Autodesk Fusion 360 part; units mm, degrees
sketch "center" plane through (0, 0, 0) normal (0, 0, 1) x (1, 0, 0)
  line L0 (3.9767, 19.6007) -> (11, 21)
  line L1 (11, 21) -> (9.3026, 17.7049)
  arc A0 (3.9767, 19.6007) -> (0, 20) centre (0, 0) ccw
  arc A1 (11.8706, 16.0962) -> (9.3026, 17.7049) centre (0, 0) ccw
  arc A2 (-8.3037, 18.1947) -> (-11.7557, 16.1803) centre (0, 0) ccw
  line L2 (-8.3037, 18.1947) -> (-3.4443, 23.455)
  line L3 (-3.4443, 23.455) -> (-2.8807, 19.7915)
  arc A3 (0.1424, 19.9995) -> (-2.8807, 19.7915) centre (0, 0) ccw
  arc A4 (-17.4124, 9.839) -> (-19.0211, 6.1803) centre (0, 0) ccw
  line L4 (-17.4124, 9.839) -> (-16.573, 16.951)
  line L5 (-16.573, 16.951) -> (-13.9637, 14.3184)
  arc A5 (-11.6402, 16.2636) -> (-13.9637, 14.3184) centre (0, 0) ccw
  arc A6 (-19.8702, -2.2748) -> (-19.0211, -6.1803) centre (0, 0) ccw
  line L6 (-19.8702, -2.2748) -> (-23.3714, 3.9723)
  line L7 (-23.3714, 3.9723) -> (-19.713, 3.3762)
  arc A7 (-18.9766, 6.3156) -> (-19.713, 3.3762) centre (0, 0) ccw
  arc A8 (-14.7382, -13.5198) -> (-11.7557, -16.1803) centre (0, 0) ccw
  line L8 (-14.7382, -13.5198) -> (-21.2427, -10.5237)
  line L9 (-21.2427, -10.5237) -> (-17.9326, -8.8556)
  arc A9 (-19.0647, -6.0447) -> (-17.9326, -8.8556) centre (0, 0) ccw
  arc A10 (-3.9767, -19.6007) -> (0, -20) centre (0, 0) ccw
  line L10 (-3.9767, -19.6007) -> (-11, -21)
  line L11 (-11, -21) -> (-9.3026, -17.7049)
  arc A11 (-11.8706, -16.0962) -> (-9.3026, -17.7049) centre (0, 0) ccw
  arc A12 (8.3037, -18.1947) -> (11.7557, -16.1803) centre (0, 0) ccw
  line L12 (8.3037, -18.1947) -> (3.4443, -23.455)
  line L13 (3.4443, -23.455) -> (2.8807, -19.7915)
  arc A13 (-0.1424, -19.9995) -> (2.8807, -19.7915) centre (0, 0) ccw
  arc A14 (17.4124, -9.839) -> (19.0211, -6.1803) centre (0, 0) ccw
  line L14 (17.4124, -9.839) -> (16.573, -16.951)
  line L15 (16.573, -16.951) -> (13.9637, -14.3184)
  arc A15 (11.6402, -16.2636) -> (13.9637, -14.3184) centre (0, 0) ccw
  arc A16 (19.8702, 2.2748) -> (19.0211, 6.1803) centre (0, 0) ccw
  line L16 (19.8702, 2.2748) -> (23.3714, -3.9723)
  line L17 (23.3714, -3.9723) -> (19.713, -3.3762)
  arc A17 (18.9766, -6.3156) -> (19.713, -3.3762) centre (0, 0) ccw
  arc A18 (14.7382, 13.5198) -> (11.7557, 16.1803) centre (0, 0) ccw
  line L18 (14.7382, 13.5198) -> (21.2427, 10.5237)
  line L19 (21.2427, 10.5237) -> (17.9326, 8.8556)
  arc A19 (19.0647, 6.0447) -> (17.9326, 8.8556) centre (0, 0) ccw
  circle A20 centre (0, 0) radius 2.75
  dimension "d248" = 40
  dimension "d250" = 360
  dimension "d253" = 5.5
extrude "Extrude13" add sketch "center" along normal blind 4
equation "StockHeight = 3 mm"
equation "d250 = C-Pattern1-Angle"
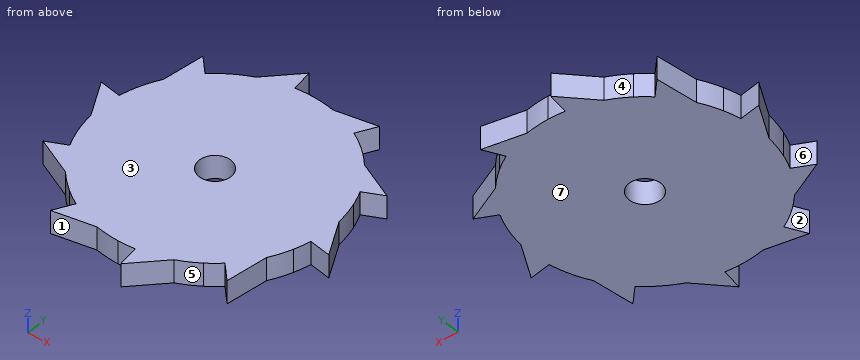
Input: part model. Units: mm. Frame: model coordinates. Face numbers are marked on the shaded views. A direction names the side the tool comes from. Give positions to 0.01 mm unless a question says otherwise; leave off trailing zeros. Loops run counter-clockwise (first coordinate to the right, second up) from the corner with the lowest first, then second, coordinate; pieces in that order, holes last. Notation, with made-up numbers: M 22.25,70.25 L 37.25,70.25 A26 cw 37.25,100.25 Z; hole C -3.75,-30.75 d6. An arc over 180 degrees is marked long. Answer as CSV lines item,"result". Start each with the question number.
1. Line query: L1, parallel to Y at x = 0, z = 1; L2, parallel to Y at x = 1.5, z = 1; L3, parallel to X at y = 15, z = 2.55. Output: solid intervals per line, ascending.
2. Pin query (flat end, axial travel): P1, Ø1.5, axis at y = 5, z = 3.5, coming from the -X side; P2, Ø1, axis at x = -13, z = 3.5, coming from the +Y side; P3, Ø1, axis at x = 18, z = 1.5, coming from the -Y side. Return the tip coordinate at first contact, or that it passes through.
3. Section A-A on y = 0. Return loops of the section in (x, z).
4. Pull-direction query (X, two-part tool) for the marked faces 5, 6 and 7; classes: released by +X, released by -X, zero draft, split by the parting line, or undercut.
5. Section B-B on x = 16. Return loops of the section in (y, z), plus the area to 3 significant figures.
6. Reachability of the marked faces 1, 2, 3 and 4 from +Z, -Z, +X, -X, +Y, -Y: full face, straight path, thin tool, end or side. Return the list, or none.
7. Section C-C on y = 11.5. Return loops of the section in (x, z), plus the area to 3 significant figures.
Computed values:
1,L1,"y = -20 to -2.75, 2.75 to 20"
1,L2,"y = -19.94 to -2.3, 2.3 to 19.94"
1,L3,"x = -16.8 to -14.64, -13.23 to 13.23"
2,P1,"stops at x = -19.54"
2,P2,"stops at y = 15.61"
2,P3,"stops at y = -9.68"
3,outline,"M -21.15,0 L -2.75,0 L -2.75,4 L -21.15,4 Z; M 2.75,0 L 21.15,0 L 21.15,4 L 2.75,4 Z"
4,face 5,"undercut"
4,face 6,"released by -X"
4,face 7,"zero draft"
5,outline,"M -16.37,0 L 12.94,0 L 12.94,4 L -16.37,4 Z"
5,area,"117 mm²"
6,face 1,"+Z, -Z, -Y"
6,face 2,"+Z, -Z, -X"
6,face 3,"+Z, +X, -X, +Y, -Y"
6,face 4,"+Z, -Z, +Y"
7,outline,"M -17.22,0 L 19.12,0 L 19.12,4 L -17.22,4 Z"
7,area,"145 mm²"
